Could you check a few things on this model? Use its own coordinates, in mm. Face numbers are marked on the shaded views. A direction names the side the tool comes from. Round coordinates to 2 decimals unless told otherwise and drop trailing zeros. Write each loop counter-clockwise with the first axis right and the second up, starting at its lowest first coordinate (ties: lowest second). Pieces come first, ordered by that corner, then holes. Notation, with made-up numbers: (47.5, 81) -> (79.5, 81) arc R6 ccw to (79.5, 85) -> close; hole circle Ø4 at (38.25, 35.25). An arc over 180 degrees is marked (long way). Answer in a Markdown table with one row per item.
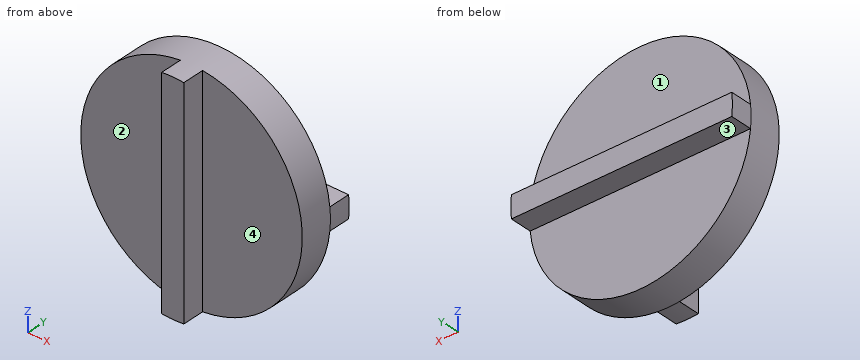
from build123d import *
from build123d.topology import SkipClean

# Parameters (mm, degrees)
SKETCH1_R           = 50
BOSS_EXTRUDE1_DEPTH = 15
BOSS_EXTRUDE2_DEPTH = 10
BOSS_EXTRUDE3_START = 10
BOSS_EXTRUDE3_DEPTH = 10


with BuildPart() as part:
    # Sketch1 → Boss-Extrude1 (new body)
    with BuildSketch(Plane(origin=(0, 0, 0), x_dir=(1, 0, 0), z_dir=(0, 1, 0))):
        with Locations(Location((0, 0, 0), (0, 0, 270))):
            Circle(SKETCH1_R)
    extrude(amount=BOSS_EXTRUDE1_DEPTH)

    # Sketch2 → Boss-Extrude2 (add)
    with SkipClean():  # the faces are left unmerged after this step: merging them gives an invalid solid
        with BuildSketch(Plane(origin=(0, 15, 0), x_dir=(1, 0, 0), z_dir=(0, 1, 0))):
            with BuildLine():
                Line((-49.749371855, 5), (49.749371855, 5))
                ThreePointArc((49.749371855, 5), (50, 0), (49.749371855, -5))
                Line((49.749371855, -5), (-49.749371855, -5))
                ThreePointArc((-49.749371855, -5), (-50, 0), (-49.749371855, 5))
            make_face()
        extrude(amount=BOSS_EXTRUDE2_DEPTH)

    # Sketch3 → Boss-Extrude3 (add)
    with SkipClean():  # the faces are left unmerged after this step: merging them gives an invalid solid
        with BuildSketch(Plane.XZ.offset(BOSS_EXTRUDE3_START)):
            with BuildLine():
                ThreePointArc((-5, -49.749371855), (0, -50), (5, -49.749371855))
                Line((5, -49.749371855), (5, 49.749371855))
                ThreePointArc((5, 49.749371855), (0, 50), (-5, 49.749371855))
                Line((-5, 49.749371855), (-5, -49.749371855))
            make_face()
        extrude(amount=-BOSS_EXTRUDE3_DEPTH)


solid = part.part
1) For the marked faces 1, 2, 3 and 4, which set-ups out of +Z, -Z, +X, -X, +Y, -Y let a thin tool reach every point of the face, with its end or its side?
Findings:
| item | result |
|---|---|
| face 1 | +Z, +X, -X, +Y |
| face 2 | +Z, -Z, -X, -Y |
| face 3 | -Z, +X, -X, +Y |
| face 4 | +Z, -Z, +X, -Y |
2) Imagine slicing it at A-A, the plane x = 0. Please give me the cut outline in (y, z), plus the area to 3 significant figures.
Findings:
| item | result |
|---|---|
| outline | (-10, -50) -> (15, -50) -> (15, -5) -> (25, -5) -> (25, 5) -> (15, 5) -> (15, 50) -> (-10, 50) -> close |
| area | 2,600 mm^2 |
3) Imagine slicing it at B-B, the plane z = 0. Please give me the cut outline in (x, y).
Findings:
| item | result |
|---|---|
| outline | (-50, 0) -> (-5, 0) -> (-5, -10) -> (5, -10) -> (5, 0) -> (50, 0) -> (50, 25) -> (-50, 25) -> close |
4) For pin 1 (2 mm diameter, centred on x = 10, z = -30.5, fed in from +Y); pin 2 (10 mm diameter, centred on x = -37.5, y = 18, fed in from -Z); pin 3 (12 mm diameter, centred on y = 12, z = 9.5, fed in from +X), each with a flat end and sliding along its axis, tell me the tip position at first contact or that it passes through.
Findings:
| item | result |
|---|---|
| pin 1 | stops at y = 15 |
| pin 2 | stops at z = -37.12 |
| pin 3 | stops at x = 49.88 |
5) Please list where these lines run through material, in increasing order: line 1 (Y direction, x = -37, z = 1); line 2 (Y direction, x = -16, z = -45); line 3 (Z direction, x = 29, y = 18.5).
Findings:
| item | result |
|---|---|
| line 1 | y = 0 to 25 |
| line 2 | y = 0 to 15 |
| line 3 | z = -5 to 5 |
6) Imagine slicing it at C-C, the plane y = -4. Please give me the cut outline in (x, z), plus the area to 3 significant figures.
Findings:
| item | result |
|---|---|
| outline | (-5, -49.75) arc R50 ccw to (5, -49.75) -> (5, 49.75) arc R50 ccw to (-5, 49.75) -> close |
| area | 998 mm^2 |
